Geometry: see drawing. Coordinates: mm, zero at the bounding-box minimum. A direction names the side the tool comes from. Coordinates: 2 decimals unless noted, no trailing zeros. Loops run counter-clockwise (first coordinate to the right, second up) from the corner with the lowest first, then second, coordinate; pieces in that order, holes last. Notation, with made-up numbers: (81, 62) - (87, 62) arc R18 ccw to (87, 73) - close; hole circle Ø6 at (-27.5, 78.5). An arc over 180 degrees is marked (long way). Answer in a Markdown table with one row per item.
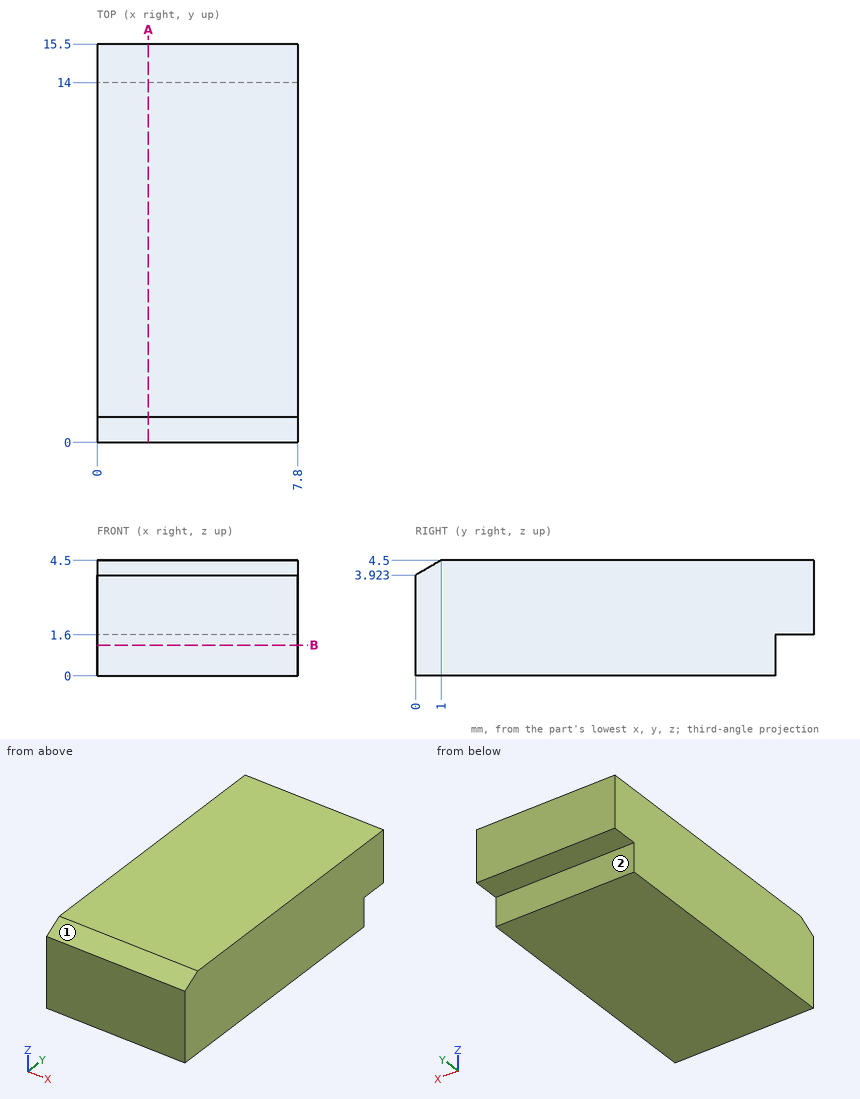
(1) Ray query, probe 1 along Y at (x, z) = (4.75, 0.65); probe 2 along Y at (x, z) = (4.5, 4.15) (1 decimal). Return the intervals inside material, ascending.
Verdict:
| item | result |
|---|---|
| probe 1 | y = 0 to 14 |
| probe 2 | y = 0.4 to 15.5 |
(2) First-contact query: pin 1 Ø0.5 at (x, z) = (2, 1) entering from +Y. Flat tip, straight axial feed; report the tip coordinate or a pass-through.
Verdict:
| item | result |
|---|---|
| pin 1 | stops at y = 14 |
(3) Cut plane A-A on x = 2. Output: boundary loops of the cut face in (y, z).
Verdict:
| item | result |
|---|---|
| outline | (0, 0) - (14, 0) - (14, 1.6) - (15.5, 1.6) - (15.5, 4.5) - (1, 4.5) - (0, 3.92) - close |
(4) Cut plane B-B on z = 1.2. Output: boundary loops of the cut face in (x, y).
Verdict:
| item | result |
|---|---|
| outline | (0, 0) - (7.8, 0) - (7.8, 14) - (0, 14) - close |
(5) Access query for the marked faces 1 and 2. Directions: +Z, -Z, +X, -X, +Y, -Y. A direction counts if a zero-diameter tool reaches every point of the face in a straight line with its end or side. Return the directions, or none.
Verdict:
| item | result |
|---|---|
| face 1 | +Z, +X, -X, -Y |
| face 2 | -Z, +X, -X, +Y |
